from build123d import *

# Parameters (mm, degrees)
SKETCH2_R                = 64.135
BOSS_EXTRUDE1_DEPTH      = 6.35
SKETCH3_R                = 64.135
SKETCH3_R_2              = 39.2557
BOSS_EXTRUDE2_DEPTH      = 50.8
SKETCH4_R                = 63.373
SKETCH4_R_2              = 39.2557
BOSS_EXTRUDE3_DEPTH      = 3.175
CUT_EXTRUDE1_DEPTH       = 61.325
FILLET1_R                = 2.54
CIRPATTERN1_COUNT        = 4
FILLET1_OF_CIRPATTERN1_R = 2.54


with BuildPart() as part:
    # Sketch2 → Boss-Extrude1 (new body)
    with BuildSketch(Plane.XY):
        Circle(SKETCH2_R)
    extrude(amount=BOSS_EXTRUDE1_DEPTH)

    # Sketch3 → Boss-Extrude2 (add)
    with BuildSketch(Plane.XY.offset(6.35)):
        Circle(SKETCH3_R)
        Circle(SKETCH3_R_2, mode=Mode.SUBTRACT)
    extrude(amount=BOSS_EXTRUDE2_DEPTH)

    # Sketch4 → Boss-Extrude3 (add)
    with BuildSketch(Plane.XY.offset(57.15)):
        Circle(SKETCH4_R)
        Circle(SKETCH4_R_2, mode=Mode.SUBTRACT)
    extrude(amount=BOSS_EXTRUDE3_DEPTH)

    # Sketch5 → Cut-Extrude1 (cut, through all)
    with BuildSketch(Plane.XY.offset(60.325)):
        with BuildLine():
            Line((-10.160122789, 37.918094459), (-16.599359458, 61.949652869))
            ThreePointArc((-16.599359458, 61.949652869), (0, 64.135), (16.599359458, 61.949652869))
            Line((16.599359458, 61.949652869), (10.160122789, 37.918094459))
            ThreePointArc((10.160122789, 37.918094459), (0, 39.2557), (-10.160122789, 37.918094459))
        make_face()
    cut_extrude1 = extrude(amount=-CUT_EXTRUDE1_DEPTH, mode=Mode.SUBTRACT)

    # Fillet1
    fillet1_edges = [part.edges().sort_by_distance(p)[0] for p in [
        (16.599359458, 61.949652869, 28.575),
        (10.160122789, 37.918094459, 33.3375),
        (-10.160122789, 37.918094459, 33.3375),
        (-16.599359458, 61.949652869, 28.575),
    ]]
    fillet(fillet1_edges, radius=FILLET1_R)

    # CirPattern1: Cut-Extrude1 ×4 about axis
    cirpattern1_axis = Axis((0, 0, 0), (0, 0, 1))
    for i in range(1, CIRPATTERN1_COUNT):
        add(cut_extrude1.rotate(cirpattern1_axis, i * 360 / CIRPATTERN1_COUNT), mode=Mode.SUBTRACT)

    # Fillet1 of CirPattern1
    fillet1_of_cirpattern1_edges = [part.edges().sort_by_distance(p)[0] for p in [
        (-61.949652869, 16.599359458, 28.575),
        (-37.918094459, 10.160122789, 33.3375),
        (-37.918094459, -10.160122789, 33.3375),
        (-61.949652869, -16.599359458, 28.575),
        (-16.599359458, -61.949652869, 28.575),
        (-10.160122789, -37.918094459, 33.3375),
        (10.160122789, -37.918094459, 33.3375),
        (16.599359458, -61.949652869, 28.575),
        (61.949652869, -16.599359458, 28.575),
        (37.918094459, -10.160122789, 33.3375),
        (37.918094459, 10.160122789, 33.3375),
        (61.949652869, 16.599359458, 28.575),
    ]]
    fillet(fillet1_of_cirpattern1_edges, radius=FILLET1_OF_CIRPATTERN1_R)


solid = part.part
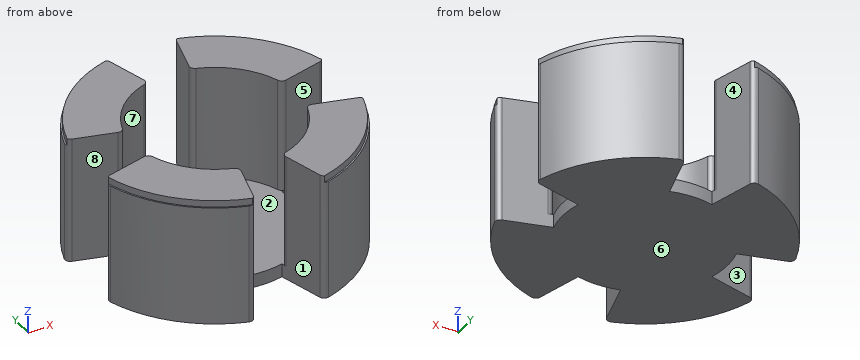
Geometry check sheet. Reference: the model listing, model coordinates, mm. Face numbers are marked on the shaded views. A direction names the side the tool comes from. Give positions to 0.01 mm unless a question says otherwise; leave off trailing zeros. Loops run counter-clockwise (first coordinate to the right, second up) from the corner with the lowest first, then second, coordinate; pieces in that order, holes last. Notation, with made-up numbers: (-30, 14.5) -> (-20, 14.5) arc R22 cw to (-20, 34.5) -> close; hole circle Ø8 at (84.25, 25). An arc over 180 degrees is marked (long way). Answer in a Markdown table with one row per item. Add a question column.
1) Cross-section at D-D on y = 31.5. Record the boundary of the cut face in (x, z) (3 decimals), and give its area (3 significant figures).
2) Cross-section at B-B on z = 8.5. State how many separate pieces and enclosed holes the cut face has, and give its area (3 significant figures).
3) Draft check along X on the marked faces 6, 7 and 8. Enter one of: pulls with the +X half, pulls with the -X half, needs draft (parallel to the pull), parting line crosses it, or undercut.
4) Cross-section at C-C on x = 54. Record the boundary of the cut face in (y, z) (3 decimals).
5) Set-up check for the marked faces 1, 2, 3, 4 and 5: record each of +Z, -Z, +X, -X, +Y, -Y from which the full face is reachable in a straight line by a thin tool's end or side.
6) Material ranges on probe 1 along Z at (x, y) = (-13, -11); probe 2 along X at (y, z) = (43.5, 57); probe 3 along X at (y, z) = (-51.5, 12.5), recorded low to high. Write a range as from..to.
7) Gauge pin test, flat ends, axial feed: P1, Ø1.5, axis at x = -40.5, z = 6.5, coming from the -Y side; P2, Ø3, axis at y = 35.5, z = 15, coming from the -X side; P3, Ø5, axis at x = -33.5, z = 29.5, coming from the -Y side. Record the tip position at first contact, or that the pin passes through.
8) Cross-section at A-A on y = 49. Record the boundary of the cut face in (x, z) (3 decimals), and give its area (3 significant figures).
Outcome:
| question | item | result |
|---|---|---|
| 1 | outline | (-55.866, 0) -> (55.866, 0) -> (55.866, 57.15) -> (54.99, 57.15) -> (54.99, 60.325) -> (23.426, 60.325) -> (23.426, 6.35) -> (-23.426, 6.35) -> (-23.426, 60.325) -> (-54.99, 60.325) -> (-54.99, 57.15) -> (-55.866, 57.15) -> close |
| 1 | area | 4,210 mm^2 |
| 2 | separate pieces | 4 |
| 2 | enclosed holes | 0 |
| 2 | area | 5,370 mm^2 |
| 3 | face 6 | needs draft |
| 3 | face 7 | undercut |
| 3 | face 8 | pulls with the -X half |
| 4 | outline | (-34.602, 0) -> (-14.469, 0) -> (-14.469, 60.325) -> (-33.168, 60.325) -> (-33.168, 57.15) -> (-34.602, 57.15) -> close; (14.469, 0) -> (34.602, 0) -> (34.602, 57.15) -> (33.168, 57.15) -> (33.168, 60.325) -> (14.469, 60.325) -> close |
| 5 | face 1 | +Z, -Z, -Y |
| 5 | face 2 | +Z |
| 5 | face 3 | +Z, -Z, -X |
| 5 | face 4 | +Z, -Z, +Y |
| 5 | face 5 | +Z, -Z, +X |
| 6 | probe 1 | z = 0..6.35 |
| 6 | probe 2 | x = -47.13..-11.66, 11.66..47.13 |
| 6 | probe 3 | x = -38.22..-13.8, 13.8..38.22 |
| 7 | P1 | stops at y = -50.33 |
| 7 | P2 | stops at x = -54.38 |
| 7 | P3 | stops at y = -56.15 |
| 8 | outline | (-41.38, 0) -> (-13.13, 0) -> (-13.13, 60.325) -> (-40.189, 60.325) -> (-40.189, 57.15) -> (-41.38, 57.15) -> close; (13.13, 0) -> (41.38, 0) -> (41.38, 57.15) -> (40.189, 57.15) -> (40.189, 60.325) -> (13.13, 60.325) -> close |
| 8 | area | 3,400 mm^2 |
